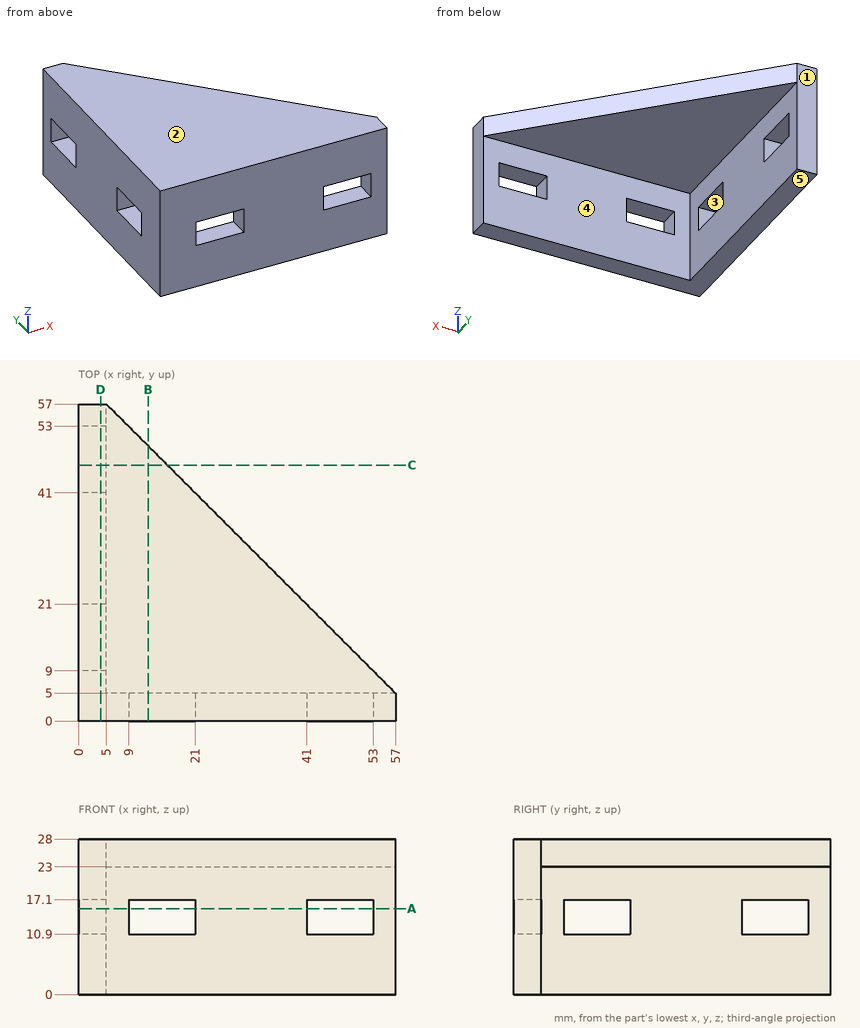
For this review, use the dimensioned drawing (mm, ordinates from the lowest corner) and the shaded views. A direction names the side the tool comes from. Coordinates: 2 decimals unless noted, no trailing zeros. Loops run counter-clockwise (first coordinate to the right, second up) from the corner with the lowest first, then second, coordinate; pieces in that order, holes last.
1. For the marked faces 4 and 5, list the 3-axis set-ups (+Z, -Z, +X, -X, +Y, -Y) from which the entire face can be reached by the end or side of a thin tool; tool diameter is ignored.
2. Insertion check: P1, Ø8, axis at y = 32, z = 9, coming from the +X side; P2, Ø6, axis at x = 13.5, z = 3, coming from the +Y side. Each pin has a flat end and moves straight along its axis. Give the tip position at first contact, or say it passes through.
3. Mouldability with a two-part tool opening along Y and no side actions: class the marked faces 1, 2 and 3 as +Y half, -Y half, draft (parallel to the pull), parting line (faces both ways), or undercut.
4. Add section B-B, the plane x = 12.5. Give the boundary of the cut face in (y, z), then the cut area to 4 significant figures.
5. Add section A-A, the plane z = 15.5. Give the boundary of the cut face in (x, y), then the cut area to 3 significant figures.
6. Add section C-C, the plane y = 46. Give the boundary of the cut face in (x, z), then the cut area to 3 significant figures.
7. Add section D-D, the plane x = 4. Give the boundary of the cut face in (y, z), then the cut area to 3 significant figures.
8. For line 1 (X direction, y = 42, z = 5.25); line 2 (Z direction, x = 21, y = 12.5), list the stretches that pass through material, from the lowest coordinate up.
Result:
1. face 4: -Z, +X, +Y
1. face 5: -Z, +X, -X, +Y, -Y
2. P1: stops at x = 5
2. P2: stops at y = 5
3. face 1: +Y half
3. face 2: draft
3. face 3: undercut
4. outline: (0, 0) - (5, 0) - (5, 10.9) - (0, 10.9) - close; (0, 17.1) - (5, 17.1) - (5, 23) - (49.5, 23) - (49.5, 28) - (0, 28) - close
4. area: 331.5 mm2
5. outline: (0, 0) - (9, 0) - (9, 5) - (5, 5) - (5, 9) - (0, 9) - close; (0, 21) - (5, 21) - (5, 41) - (0, 41) - close; (0, 53) - (5, 53) - (5, 57) - (0, 57) - close; (21, 0) - (41, 0) - (41, 5) - (21, 5) - close; (53, 0) - (57, 0) - (57, 5) - (53, 5) - close
5. area: 305 mm2
6. outline: (0, 0) - (5, 0) - (5, 10.9) - (0, 10.9) - close; (0, 17.1) - (5, 17.1) - (5, 23) - (16, 23) - (16, 28) - (0, 28) - close
6. area: 164 mm2
7. outline: (0, 0) - (57, 0) - (57, 28) - (0, 28) - close; hole (9, 10.9) - (21, 10.9) - (21, 17.1) - (9, 17.1) - close; hole (41, 10.9) - (53, 10.9) - (53, 17.1) - (41, 17.1) - close
7. area: 1,450 mm2
8. line 1: x = 0 to 5
8. line 2: z = 23 to 28
